Source: CAD feature listing. Evaluate the final solid. Frame: model axes, mm. A direction names the side the tool comes from. Give positions to 0.01 mm unless a question says otherwise; leave off trailing zeros. Loops run counter-clockwise (first coordinate to the right, second up) from the corner with the lowest first, then second, coordinate; pieces in that order, holes last. Notation, with made-up numbers: (61.5, 17.25) - (90.5, 17.25) arc R22 ccw to (90.5, 44.25) - close; hole circle Ø9 at (35.25, -21.5). An arc over 180 degrees is marked (long way). Put each result on its own line as item: value.
Autodesk Inventor part; units mm, degrees
ref_plane "作業平面1" through (19.45, -4.102, -7.5) normal (0, 0, 1) x (1, 0, 0)
ref_plane "YZ Plane" through (0, 0, 0) normal (1, 0, 0) x (0, 1, 0)
ref_plane "XZ Plane" through (0, 0, 0) normal (0, 1, 0) x (-1, 0, 0)
sketch "スケッチ1" plane through (0, 0, 0) normal (0, 0, 1) x (1, 0, 0)
  circle A0 centre (0, 12.3) radius 0.8
  circle A1 centre (0, -12.3) radius 0.8
  line L0 (-4, -13.8) -> (4, -13.8)
  line L1 (4, -13.8) -> (4, 13.8)
  line L2 (4, 13.8) -> (-4, 13.8)
  line L3 (-4, 13.8) -> (-4, -13.8)
  line L4 (-4, -13.8) -> (4, 13.8) construction
  line L5 (4, -13.8) -> (-4, 13.8) construction
  point P0 (0, 0)
  dimension "d0" = 1.6
  dimension "d1" = 24.6
  dimension "d2" = 12.3
  dimension "d3" = 1.5
  dimension "d4" = 4
extrude "押し出し1" add sketch "スケッチ1" along normal blind 3
sketch "スケッチ2" plane through (0, 0, 3) normal (0, 0, 1) x (1, 0, 0)
  circle A0 centre (21.45, 3.898) radius 0.55
  line L0 (19.45, 5.898) -> (19.45, -4.102)
  line L1 (19.45, -4.102) -> (23.45, -4.102)
  line L2 (23.45, -4.102) -> (23.45, 5.898)
  line L3 (23.45, 5.898) -> (19.45, 5.898)
  line L4 (23.45, -4.102) -> (4, -4.102)
  line L5 (4, -4.102) -> (4, 5.898)
  line L6 (4, 5.898) -> (23.45, 5.898)
  line L7 (23.45, 5.898) -> (23.45, -4.102)
  line L8 (4, -13.8) -> (4, 13.8)
  point P0 (0, 0)
extrude "押し出し2" add sketch "スケッチ2" against normal up to surface (3 mm away)
sketch "スケッチ3" plane through (0, 0, 0) normal (0, 0, -1) x (-1, 0, 0)
  circle A0 centre (-21.45, 3.898) radius 0.55
  line L0 (-19.45, 5.898) -> (-19.45, -4.102)
  line L1 (-19.45, -4.102) -> (-23.45, -4.102)
  line L2 (-23.45, -4.102) -> (-23.45, 5.898)
  line L3 (-23.45, 5.898) -> (-19.45, 5.898)
  point P0 (0, 0)
ref_plane "作業平面1" through (19.45, -4.102, -7.5) normal (0, 0, 1) x (1, 0, 0)
extrude "押し出し3" add sketch "スケッチ3" along normal up to surface (7.5 mm away)
sketch "スケッチ4" plane through (0, 0, 3) normal (0, 0, 1) x (1, 0, 0)
  line L0 (23.45, -4.102) -> (23.45, 5.898)
  line L1 (19.45, 5.898) -> (19.45, -4.102)
  line L2 (23.45, 5.898) -> (19.45, 5.898)
  line L3 (19.45, 5.898) -> (19.45, 1.398)
  line L4 (19.45, 1.398) -> (23.45, 1.398)
  line L5 (23.45, 1.398) -> (23.45, 5.898)
  point P0 (0, 0)
  dimension "d11" = 4.5
extrude "押し出し4" cut sketch "スケッチ4" against normal blind 8
fillet "フィレット1" radius 2 4 edges at (4, -13.8, 1.5) (-4, -13.8, 1.5) (4, 13.8, 1.5) (-4, 13.8, 1.5)
move faces "移動1" translate (0, 0, -1) faces at (-1.3333, -1.3673, 3)
sketch "スケッチ5" plane through (4, -4.102, 2) normal (0, 0, 1) x (1, 0, 0)
  line L0 (15.45, 10) -> (0, 10)
  line L1 (0, 10) -> (-8, 10)
  line L2 (-8, 10) -> (-8, 17.902)
  line L3 (-8, 17.902) -> (0, 17.902)
  line L4 (0, 17.902) -> (0, 10)
  point P0 (-4, 4.102)
  point P1 (-8, 15.902)
  point P2 (-6, 17.902)
extrude "押し出し5" cut sketch "スケッチ5" against normal through all
fillet "フィレット2" radius 2 2 edges at (4, -4.102, 1) (-4, 5.898, 1)
properties part number "HbServoCover"
1) Section query D-D, the plane y = -2. Output: boundary loops of the cut face in (x, z), plus the area to 3 significant figures.
Check result:
outline: (-4, 0) - (19.45, 0) - (19.45, -7.5) - (23.45, -7.5) - (23.45, 2) - (-4, 2) - close
area: 84.9 mm²
2) Access query for faces 4 (the flat face through (4, -9, 1)), 5 (the flat face through (19.45, 0, -5)), 6 (the flat face through (21, 3, -5)), 7 (the flat face through (21, 1.398, -1)). Directions: +Z, -Z, +X, -X, +Y, -Y. A direction counts if a zero-diameter tool reaches every point of the face in a straight line with its end or side. Return the directions, or none.
Check result:
face 4: +Z, -Z, +X, -Y
face 5: -Z, -X, +Y, -Y
face 6: +Z, +X, -X, +Y
face 7: +Z, +X, +Y
3) Mould query, pull axis Y, two halves, no side actions, for faces 1 (the flat face through (6, -2, 2)), 2 (the cylindrical face through (-0.104, -13.093, 0.986)), 3 (the flat face through (21, 5.898, -6)). Classes: pulls with the +Y half, pulls with the -Y half, needs draft (parallel to the pull), parting line crosses it, or undercut.
Check result:
face 1: needs draft
face 2: undercut
face 3: pulls with the +Y half
4) Section query C-C, the plane y = -12.3. Output: boundary loops of the cut face in (x, z), plus the area to 3 significant figures.
Check result:
outline: (-3.94, 0) - (-0.8, 0) - (-0.8, 2) - (-3.94, 2) - close; (0.8, 0) - (3.94, 0) - (3.94, 2) - (0.8, 2) - close
area: 12.5 mm²
5) Section query A-A, the plane x = 0. Output: boundary loops of the cut face in (y, z).
Check result:
outline: (-13.8, 0) - (-13.1, 0) - (-13.1, 2) - (-13.8, 2) - close; (-11.5, 0) - (5.9, 0) - (5.9, 2) - (-11.5, 2) - close
6) Material intervals for line 1 along Y through (x, z) = (21.45, -6.8); line 2 along X through (y, z) = (4.75, -5.5); line 3 along Z through (x, y) = (14.5, 5), sorted ascending. Write a range as [from, to].
Check result:
line 1: [-4.1, 3.35], [4.45, 5.9]
line 2: [19.45, 23.45]
line 3: [0, 2]
7) Pin query (flat end, axial travel): P1, Ø1.8, axis at x = 0, y = -12.3, coming from the -Z side; P2, Ø3, axis at x = 22.5, y = 4, coming from the +Z side; P3, Ø1.6, axis at y = 4, z = 1, coming from the +X side. Return the tip coordinate at first contact, or that it passes through.
Check result:
P1: z = 0
P2: z = -5
P3: x = 19.45
8) Section query B-B, the plane z = -6. Output: boundary loops of the cut face in (x, y), plus the area to 3 significant figures.
Check result:
outline: (19.45, -4.1) - (23.45, -4.1) - (23.45, 5.9) - (19.45, 5.9) - close; hole circle Ø1.1 at (21.45, 3.9)
area: 39.0 mm²
